```python
from build123d import *

# Parameters (mm, degrees)
SKETCH_W        = 63
SKETCH_H        = 114
SKETCH_R        = 1.95
SKETCH_R_2      = 5.525
SKETCH_R_3      = 1.6
PAD_DEPTH       = 10
SKETCH004_R     = 11.525
PAD001_DEPTH    = 3
SKETCH003_R     = 5.55
POCKET_DEPTH    = 13.001
SKETCH006_R     = 11
POCKET001_DEPTH = 3
SKETCH007_R     = 3.5
POCKET002_DEPTH = 0.01
POCKET003_DEPTH = 10.001
SKETCH009_R     = 1.7
POCKET004_DEPTH = 12
PAD002_DEPTH    = 13
PAD003_DEPTH    = 6
SKETCH023_R     = 2.75
POCKET005_DEPTH = 9
SKETCH025_R     = 2
POCKET006_DEPTH = 16
SKETCH026_R     = 6
POCKET007_DEPTH = 2


with BuildPart() as part:
    # Sketch → Pad (new body)
    with BuildSketch(Plane.XY):
        with Locations((-1.5, -29)):
            Rectangle(SKETCH_W, SKETCH_H)
        with Locations((-15.5, 15.5)):
            Circle(SKETCH_R, mode=Mode.SUBTRACT)
        with Locations((15.5, 15.5)):
            Circle(SKETCH_R, mode=Mode.SUBTRACT)
        with Locations((-15.5, -15.5)):
            Circle(SKETCH_R, mode=Mode.SUBTRACT)
        with Locations((15.5, -15.5)):
            Circle(SKETCH_R, mode=Mode.SUBTRACT)
        with Locations((0, -58)):
            Circle(SKETCH_R_2, mode=Mode.SUBTRACT)
        with Locations((-15.5, -42.5)):
            Circle(SKETCH_R_3, mode=Mode.SUBTRACT)
        with Locations((15.5, -42.5)):
            Circle(SKETCH_R_3, mode=Mode.SUBTRACT)
        with Locations((-15.5, -73.5)):
            Circle(SKETCH_R_3, mode=Mode.SUBTRACT)
        with Locations((15.5, -73.5)):
            Circle(SKETCH_R_3, mode=Mode.SUBTRACT)
    extrude(amount=PAD_DEPTH)

    # Sketch004 (on Face15 of Pad) → Pad001 (join)
    with BuildSketch(Plane.XY.offset(10)):
        Circle(SKETCH004_R)
    extrude(amount=PAD001_DEPTH)

    # Sketch003 (on Face17 of Pad001) → Pocket (cut, through all)
    with BuildSketch(Plane.XY.offset(13)):
        Circle(SKETCH003_R)
    extrude(amount=-POCKET_DEPTH, mode=Mode.SUBTRACT)

    # Sketch006 (on Face5 of Pocket) → Pocket001 (cut)
    with BuildSketch(Plane.XY.offset(10)):
        with Locations((0, -58)):
            Circle(SKETCH006_R)
    extrude(amount=-POCKET001_DEPTH, mode=Mode.SUBTRACT)

    # Sketch007 (on Face4 of Pocket001) → Pocket002 (cut)
    with BuildSketch(Plane(origin=(0, 0, 0), x_dir=(1, 0, 0), z_dir=(0, 0, -1))):
        with Locations((-15.5, 73.5)):
            Circle(SKETCH007_R)
        with Locations((15.5, 73.5)):
            Circle(SKETCH007_R)
        with Locations((15.5, 42.5)):
            Circle(SKETCH007_R)
        with Locations((-15.5, 42.5)):
            Circle(SKETCH007_R)
    extrude(amount=-POCKET002_DEPTH, mode=Mode.SUBTRACT)

    # Sketch008 (on Face5 of Pocket002) → Pocket003 (cut, through all)
    with BuildSketch(Plane.XY.offset(10)):
        with BuildLine():
            ThreePointArc((-18, -28.4), (-20.6, -31), (-18, -33.6))
            Line((-18, -33.6), (-7, -33.6))
            ThreePointArc((-7, -33.6), (-4.4, -31), (-7, -28.4))
            Line((-18, -28.4), (-7, -28.4))
        make_face()
    extrude(amount=-POCKET003_DEPTH, mode=Mode.SUBTRACT)

    # Sketch009 (on Face2 of Pocket003) → Pocket004 (cut)
    with BuildSketch(Plane(origin=(-33, 0, 0), x_dir=(0, -1, 0), z_dir=(-1, 0, 0))):
        with Locations((31, 5)):
            Circle(SKETCH009_R)
    extrude(amount=-POCKET004_DEPTH, mode=Mode.SUBTRACT)

    # Sketch014 (on Face5 of Pocket004) → Pad002 (join)
    with BuildSketch(Plane.XY.offset(10)):
        Polygon((-33, 5.5), (-23, 5.5), (-23, -80), (23, -80), (23, -13.5), (30, -13.5), (30, -86), (-33, -86), align=None)
    extrude(amount=PAD002_DEPTH)

    # Sketch022 (on Face2 of Pad002) → Pad003 (join)
    with BuildSketch(Plane(origin=(-33, 0, 0), x_dir=(0, -1, 0), z_dir=(-1, 0, 0))):
        Polygon((-28, 0), (-28, 50), (-8, 50), (86, 23), (86, 0), align=None)
    extrude(amount=PAD003_DEPTH)

    # Sketch023 (on Face9 of Pad003) → Pocket005 (cut)
    with BuildSketch(Plane(origin=(-39, 0, 0), x_dir=(0, -1, 0), z_dir=(-1, 0, 0))):
        with Locations((-18, 43)):
            Circle(SKETCH023_R)
    extrude(amount=-POCKET005_DEPTH, mode=Mode.SUBTRACT)

    # Sketch025 (on Face4 of Pocket005) → Pocket006 (cut)
    with BuildSketch(Plane(origin=(0, 0, 0), x_dir=(1, 0, 0), z_dir=(0, 0, -1))):
        with Locations((26.5, -19.5)):
            Circle(SKETCH025_R)
        with Locations((-26.5, -19.5)):
            Circle(SKETCH025_R)
    extrude(amount=-POCKET006_DEPTH, mode=Mode.SUBTRACT)

    # Sketch026 (on Face5 of Pocket006) → Pocket007 (cut)
    with BuildSketch(Plane.XY.offset(10)):
        with Locations((-26.5, 19.5)):
            Circle(SKETCH026_R)
        with BuildLine():
            ThreePointArc((20.5, 19.5), (22.257359, 15.257359), (26.5, 13.5))
            Line((26.5, 13.5), (46.5, 13.5))
            Line((20.5, 46.38), (46.5, 13.5))
            Line((20.5, 46.38), (20.5, 19.5))
        make_face()
    extrude(amount=-POCKET007_DEPTH, mode=Mode.SUBTRACT)


solid = part.part
```
The model under review builds one solid part; all positions refer to its coordinate system, in mm. A direction names the side the tool comes from. Round coordinates to 2 decimals unless told otherwise and drop trailing zeros. Order: outer loops, then holes, each group sorted by start corner. A loop starts at its lowest first (then second) coordinate and runs counter-clockwise, first axis right, second up. Notation, with made-up numbers: (5.25, 68) -> (28.25, 68) arc R13 cw to (28.25, 75) -> close; hole circle Ø6 at (29.5, 70). An arc over 180 degrees is marked (long way). Use a Markdown table: item, result.
Q1. We need section A-A on y = -15.5. Write out the cut boundary in (x, z).
Values:
| item | result |
|---|---|
| outline | (-39, 0) -> (-17.45, 0) -> (-17.45, 10) -> (-23, 10) -> (-23, 23) -> (-33, 23) -> (-33, 43.25) -> (-39, 43.25) -> close; (-13.55, 0) -> (13.55, 0) -> (13.55, 10) -> (-13.55, 10) -> close; (17.45, 0) -> (30, 0) -> (30, 23) -> (23, 23) -> (23, 10) -> (17.45, 10) -> close |
Q2. We need section C-C on y = -60.5. Write out the cut boundary in (x, z), then the cut area to 3 significant figures.
Values:
| item | result |
|---|---|
| outline | (-39, 0) -> (-4.93, 0) -> (-4.93, 7) -> (-10.71, 7) -> (-10.71, 10) -> (-23, 10) -> (-23, 23) -> (-33, 23) -> (-33, 30.32) -> (-39, 30.32) -> close; (4.93, 0) -> (30, 0) -> (30, 23) -> (23, 23) -> (23, 10) -> (10.71, 10) -> (10.71, 7) -> (4.93, 7) -> close |
| area | 900 mm^2 |
Q3. Clearance check with flat-ended pins moving along their axes: P1, Ø10, axis at x = 16.5, y = 14, coming from the +Z side; P2, Ø5, axis at x = 26.5, y = 19.5, coming from the +Z side; P3, Ø1.6, axis at x = 27.5, z = 9, coming from the +Y side; P4, Ø19, axis at x = -26.5, y = 19.5, coming from the +Z side. State where each tip first meets the part, or that it passes through.
Values:
| item | result |
|---|---|
| P1 | stops at z = 10 |
| P2 | stops at z = 8 |
| P3 | stops at y = 13.5 |
| P4 | stops at z = 50 |
Q4. For line 1 (X direction, y = -56.5, z = 21.5); line 2 (Z direction, x = -29, y = -31); line 3 (X direction, y = -73, z = 3), list the stretches that pass through material, from the lowest coordinate up.
Values:
| item | result |
|---|---|
| line 1 | x = -39 to -23, 23 to 30 |
| line 2 | z = 0 to 3.3, 6.7 to 23 |
| line 3 | x = -39 to -17.02, -13.98 to 13.98, 17.02 to 30 |
Q5. We need section D-D on z = 5. State how many separate pieces and enclosed holes the cut face has, then the cut area to 3 significant figures.
Values:
| item | result |
|---|---|
| separate pieces | 1 |
| enclosed holes | 14 |
| area | 7,450 mm^2 |
Q6. Mouldability with a two-part tool opening along Z and no side actions: class faces 5 (the flat face through (5, 3, 13)), 6 (the flat face through (-39, -17, 20)), 7 (the flat face through (-21, -31, 5)) as +Z half, -Z half, draft (parallel to the pull), parting line (faces both ways), or undercut.
Values:
| item | result |
|---|---|
| face 5 | +Z half |
| face 6 | draft |
| face 7 | undercut |
Q7. We need section B-B on z = 43. Write out the cut boundary in (x, y), then the cut area to 3 significant figures.
Values:
| item | result |
|---|---|
| outline | (-39, -16.37) -> (-33, -16.37) -> (-33, 15.25) -> (-39, 15.25) -> close; (-39, 20.75) -> (-33, 20.75) -> (-33, 28) -> (-39, 28) -> close |
| area | 233 mm^2 |
Q8. Tool access review of faces 1 (the cylindrical face through (-27.08, -32.57, 4.35)), 2 (the flat face through (0, -80, 16)), 3 (the flat face through (-13, -28.4, 5)), 4 (the flat face through (-23, -37, 16)): name each direction out of +Z, -Z, +X, -X, +Y, -Y from which nothing blocks a thin tool from reaching the whole face with its end or side.
Values:
| item | result |
|---|---|
| face 1 | none |
| face 2 | +Z |
| face 3 | +Z, -Z |
| face 4 | +Z, +Y |
